Autodesk Inventor part; units mm, degrees
ref_plane "YZ Plane" through (0, 0, 0) normal (1, 0, 0) x (0, 1, 0)
ref_plane "XZ Plane" through (0, 0, 0) normal (0, 1, 0) x (-1, 0, 0)
ref_plane "XY Plane" through (0, 0, 0) normal (0, 0, 1) x (1, 0, 0)
sketch "Sketch1" plane through (0, 0, 0) normal (0, 1, 0) x (-1, 0, 0)
  line L0 (8.8039, 17.4877) -> (-8.8039, 17.4877)
  line L1 (-8.8039, 17.4877) -> (-8.8039, -17.4877)
  line L2 (-8.8039, -17.4877) -> (8.8039, -17.4877)
  line L3 (8.8039, -17.4877) -> (8.8039, 17.4877)
  line L4 (8.8039, 17.4877) -> (-8.8039, -17.4877) construction
  line L5 (-8.8039, 17.4877) -> (8.8039, -17.4877) construction
  point P0 (0, 0)
extrude "Extrusion1" add sketch "Sketch1" along normal blind 12.7
shell "Shell1" thickness 2.54 removed faces 1 at (2.9346, 12.7, 5.8292)
properties part number "BOX"
CAD build for the part. Positions are in the model's coordinates, mm. A direction names the side the tool comes from. Round coordinates to 2 decimals unless told otherwise and drop trailing zeros. Order: outer loops, then holes, each group sorted by start corner. A loop starts at its lowest first (then second) coordinate and runs counter-clockwise, first axis right, second up. Notation, with made-up numbers: (-1.75, 58.25) -> (35.25, 58.25) arc R21 cw to (35.25, 88.25) -> close; hole circle Ø6 at (63.5, 5). An arc over 180 degrees is marked (long way). Write item = value, one per line. Start each with the question number.
(1) Pin check, flat tip, straight feed: P1, Ø10, axis at x = 0, z = 7, coming from the +Y side. Stop position of the tip, or through.
(2) Which spindle directions (+Z, -Z, +X, -X, +Y, -Y) get a long thin tool onto all of the face, cutting with end or side? Do faces 1 (the flat face through (0, 8, -14.948)), 2 (the flat face through (0, 6, -17.488)). Say none if no direction does.
(3) Probe line 1 (Z direction, x = 1, y = 3); line 2 (X direction, y = 11, z = -8); line 3 (Y direction, x = 5, z = 0). List the from-to ranges inside material, lowest first. Write a range as [from, to].
(4) Cut at B-B, the plane z = -10. List the corners of the cut face in (x, y).
(5) Cut at A-A, the plane y = 9.5. List the corners of the cut face in (x, z).
(6) Cut at C-C, the plane x = -3.75. List the corners of the cut face in (y, z).
(7) Pull direction X, two halves, no side cores. Call faces 3 (the flat face through (-6.264, 8, 0)), 4 (the flat face through (8.804, 6, 0)), 5 (the flat face through (-8, 12.7, 0)): released by +X, released by -X, zero draft, split by the parting line, or undercut.
Model answer:
q1.P1 = 2.54
q2.face_1 = +Y
q2.face_2 = -Z, +X, -X, +Y, -Y
q3.line_1 = [-17.49, -14.95], [14.95, 17.49]
q3.line_2 = [-8.8, -6.26], [6.26, 8.8]
q3.line_3 = [0, 2.54]
q4.outline = (-8.8, 0) -> (8.8, 0) -> (8.8, 12.7) -> (6.26, 12.7) -> (6.26, 2.54) -> (-6.26, 2.54) -> (-6.26, 12.7) -> (-8.8, 12.7) -> close
q5.outline = (-8.8, -17.49) -> (8.8, -17.49) -> (8.8, 17.49) -> (-8.8, 17.49) -> close; hole (-6.26, -14.95) -> (6.26, -14.95) -> (6.26, 14.95) -> (-6.26, 14.95) -> close
q6.outline = (0, -17.49) -> (12.7, -17.49) -> (12.7, -14.95) -> (2.54, -14.95) -> (2.54, 14.95) -> (12.7, 14.95) -> (12.7, 17.49) -> (0, 17.49) -> close
q7.face_3 = undercut
q7.face_4 = released by +X
q7.face_5 = zero draft
